from build123d import *

# Parameters (mm, degrees)
SKETCH4_W               = 104
SKETCH4_H               = 104
BOSS_EXTRUDE2_DEPTH     = 57.5
BOSS_EXTRUDE2_TAPER     = 23
SKETCH6_R               = 25
CUT_EXTRUDE1_DEPTH      = 179.5
CUT_EXTRUDE_THIN1_START = 10
CUT_EXTRUDE_THIN1_DEPTH = 10
CUT_EXTRUDE3_DEPTH      = 124
SKETCH10_R              = 35
CUT_EXTRUDE4_DEPTH      = 10
FILLET9_R               = 15
FILLET10_R              = 15


with BuildPart() as part:
    # Sketch4 → Boss-Extrude2 (new body)
    with BuildSketch(Plane.XY):
        with Locations((52, 52)):
            Rectangle(SKETCH4_W, SKETCH4_H)
    boss_extrude2 = extrude(amount=BOSS_EXTRUDE2_DEPTH, taper=BOSS_EXTRUDE2_TAPER)

    # Mirror2: Boss-Extrude2 across plane
    add(boss_extrude2.mirror(Plane(origin=(0, 0, 57.5), x_dir=(1, 0, 0), z_dir=(0, 0, -1))))

    # Sketch6 → Cut-Extrude1 (cut)
    with BuildSketch(Plane.XY.offset(115)):
        with Locations((52, 52)):
            Circle(SKETCH6_R)
    extrude(amount=-CUT_EXTRUDE1_DEPTH, mode=Mode.SUBTRACT)

    # Sketch8 → Cut-Extrude-Thin1 (cut)
    with BuildSketch(Plane.XY.offset(CUT_EXTRUDE_THIN1_START)):
        with BuildLine():
            ThreePointArc((52, 17), (76.748737342, 76.748737342), (17, 52))
            Line((17, 52), (7, 52))
            ThreePointArc((7, 52), (83.819805153, 83.819805153), (52, 7))
            Line((52, 7), (52, 17))
        make_face()
        with BuildLine():
            ThreePointArc((52, 27), (69.67766953, 69.67766953), (27, 52))
            Line((27, 52), (17, 52))
            ThreePointArc((17, 52), (76.748737342, 76.748737342), (52, 17))
            Line((52, 17), (52, 27))
        make_face()
    extrude(amount=-CUT_EXTRUDE_THIN1_DEPTH, mode=Mode.SUBTRACT)

    # Sketch9 → Cut-Extrude3 (cut)
    with BuildSketch(Plane(origin=(0, 0, 0), x_dir=(-1, 0, 0), z_dir=(0, 0, -1))):
        Polygon((-27, 52), (0, 52), (0, 0), (-52, 0), (-52, 27), (-52, 52), align=None)
    extrude(amount=-CUT_EXTRUDE3_DEPTH, mode=Mode.SUBTRACT)

    # Sketch10 → Cut-Extrude4 (cut)
    with BuildSketch(Plane.XY.offset(115)):
        with Locations((52, 52)):
            Circle(SKETCH10_R)
    extrude(amount=-CUT_EXTRUDE4_DEPTH, mode=Mode.SUBTRACT)

    # Fillet9
    fillet9_edges = [part.edges().sort_by_distance(p)[0] for p in [
        (65.796349034, 24.407301932, 57.5),
    ]]
    fillet(fillet9_edges, radius=FILLET9_R)

    # Fillet10
    fillet10_edges = [part.edges().sort_by_distance(p)[0] for p in [
        (24.407301932, 65.796349034, 57.5),
        (52, 79.592698068, 57.5),
        (79.592698068, 51.352297169, 57.5),
    ]]
    fillet(fillet10_edges, radius=FILLET10_R)


solid = part.part
Input: part model. Units: mm. Frame: model coordinates. A direction names the side the tool comes from. Give positions to 0.01 mm unless a question says otherwise; leave off trailing zeros. Write each loop counter-clockwise with the first axis right and the second up, starting at its lowest first coordinate (ties: lowest second). Pieces come first, ordered by that corner, then holes. Notation, with made-up numbers: M 64.5,-11 L 108.5,-11 A33 cw 108.5,26 Z; hole C 60,-7 d8. An arc over 180 degrees is marked long. Write item = value, one per line. Start each with the question number.
1) Cut plane B-B on z = 88. Return the cut outline in (x, y), then the cut area to 3 significant figures.
2) Reachability of faces 1 (the cylindrical face through (82.753, 84.852, 5.07)), 2 (the flat face through (93.194, 52.728, 89.542)), 3 (the flat face through (22, 52, 69)) from +Z, -Z, +X, -X, +Y, -Y: full face, straight path, thin tool, end or side. Return the list, or none.
3) Material intervals for line 1 along Z through (x, y) = (98.5, 69); line 2 along Z through (x, y) = (95, 73); line 3 along Y through (x, z) = (50, 22.5), sorted ascending. Write a range as [from, to].
4) First-contact query: pin 1 Ø12 at (y, z) = (29.5, 44.5) entering from -X; pin 2 Ø12 at (x, z) = (86.5, 19) entering from +Y; pin 3 Ø4 at (x, z) = (71, 44.5) entering from -Y. Flat tips, straight axial feed; report the tip coordinate or a pass-through.
5) Draft query along Y for faces 4 (the flat face through (72.586, 10.806, 25.458)), 5 (the flat face through (51.272, 93.194, 89.542)), 6 (the flat face through (70, 70, 105)). Return one class per face: +Y half, -Y half, draft (parallel to the pull), parting line (faces both ways), or undercut.
6) Cut plane A-A on y = 11.5. Return the cut outline in (x, z).
7) Cut plane C-C on z = 60. Return the cut outline in (x, y).
Solved:
q1.outline = M 11.46,52 L 27,52 A25 cw long 52,27 L 52,11.46 L 92.54,11.46 L 92.54,92.54 L 11.46,92.54 Z
q1.area = 3,460 mm2
q2.face_1 = -Z
q2.face_2 = +X, +Y, -Y
q2.face_3 = +Z, -Z, -X, -Y
q3.line_1 = [0, 12.96], [102.04, 115]
q3.line_2 = [0, 21.2], [93.8, 115]
q3.line_3 = [76.92, 94.45]
q4.pin_1 = 52
q4.pin_2 = 98.48
q4.pin_3 = 18.04
q5.face_4 = -Y half
q5.face_5 = +Y half
q5.face_6 = undercut
q6.outline = M 52,10 L 71.62,10 L 71.62,0 L 104,0 L 92.5,27.09 L 52,27.09 Z; M 52,87.91 L 92.5,87.91 L 104,115 L 52,115 Z
q7.outline = M 22.9,52 L 27,52 A25 cw long 52,27 L 52,22.9 L 81.1,22.9 L 81.1,81.1 L 22.9,81.1 Z
